from build123d import *

# Parameters (mm, degrees)
SKETCH032_W            = 103
SKETCH032_H            = 207
PAD009_DEPTH           = 18
POCKET017_DEPTH        = 16
SKETCH034_W            = 55
SKETCH034_H            = 79
POCKET018_DEPTH        = 16
POCKET019_DEPTH        = 16
LINEARPATTERN002_COUNT = 3
LINEARPATTERN002_PITCH = 24
POCKET020_DEPTH        = 16
POCKET021_DEPTH        = 16
FILLET008_R            = 8
FILLET009_R            = 15
POCKET022_DEPTH        = 5
POCKET022_DEPTH_BACK   = 100


with BuildPart() as part:
    # Sketch032 → Pad009 (new body)
    with BuildSketch(Plane.XY):
        Rectangle(SKETCH032_W, SKETCH032_H)
    extrude(amount=PAD009_DEPTH)

    # Sketch029 (on Face6 of Pad009) → Pocket017 (cut)
    with BuildSketch(Plane(origin=(10, 69, 18), x_dir=(1, 0, 0), z_dir=(0, 0, 1))):
        Polygon((-40, -32), (40, -32), (40, 32), (-40, 32), (-56, 32), (-56, 16), (-40, 16), align=None)
    extrude(amount=-POCKET017_DEPTH, mode=Mode.SUBTRACT)

    # Sketch034 → Pocket018 (cut)
    with BuildSketch(Plane(origin=(-52, 30, 18), x_dir=(0, 1, 0), z_dir=(0, 0, 1))):
        with Locations((-22, -62)):
            Rectangle(SKETCH034_W, SKETCH034_H)
    extrude(amount=-POCKET018_DEPTH, mode=Mode.SUBTRACT)

    # Sketch030 → Pocket019 (cut)
    with BuildSketch(Plane(origin=(25, -90, 18), x_dir=(1, 0, 0), z_dir=(0, 0, 1))):
        with BuildLine():
            Line((-23.5, 11), (23.5, 11))
            Line((23.5, 11), (15.797717, 0))
            Line((15.797717, 0), (23.5, -11))
            Line((23.5, -11), (-23.5, -11))
            ThreePointArc((-23.5, 11), (-34.5, 0), (-23.5, -11))
        make_face()
    pocket019 = extrude(amount=-POCKET019_DEPTH, mode=Mode.SUBTRACT)

    # LinearPattern002: Pocket019 ×3
    with Locations(*[(0, i * LINEARPATTERN002_PITCH, 0) for i in range(1, LINEARPATTERN002_COUNT)]):
        add(pocket019, mode=Mode.SUBTRACT)

    # Sketch031 → Pocket020 (cut)
    with BuildSketch(Plane(origin=(-68, -55, 18), x_dir=(1, 0, 0), z_dir=(0, 0, 1))):
        with BuildLine():
            Line((51.488981, 23.283394), (51.488981, -34.716606))
            Line((51.488981, -34.716606), (46.488981, -34.716606))
            ThreePointArc((27.488981, -34.716606), (36.988981, -44.216606), (46.488981, -34.716606))
            Line((27.488981, -34.716606), (22.488981, -34.716606))
            Line((22.488981, -34.716606), (22.488981, 23.283394))
            Line((22.488981, 23.283394), (51.488981, 23.283394))
        make_face()
    extrude(amount=-POCKET020_DEPTH, mode=Mode.SUBTRACT)

    # Sketch033 → Pocket021 (cut)
    with BuildSketch(Plane(origin=(-60, 120, 18), x_dir=(1, 0, 0), z_dir=(0, 0, 1))):
        with BuildLine():
            ThreePointArc((10.250873, -136.6297), (19.384811, -145.763638), (28.518749, -136.6297))
            Line((28.518749, -136.6297), (28.518749, -47.133303))
            ThreePointArc((28.518749, -47.133303), (19.384811, -37.999364), (10.250873, -47.133303))
            Line((10.250873, -136.6297), (10.250873, -47.133303))
        make_face()
    extrude(amount=-POCKET021_DEPTH, mode=Mode.SUBTRACT)

    # Fillet008
    fillet008_edges = [part.edges().sort_by_distance(p)[0] for p in [
        (-40.615189, 82.000636, 2),
    ]]
    fillet(fillet008_edges, radius=FILLET008_R)

    # Fillet009
    fillet009_edges = [part.edges().sort_by_distance(p)[0] for p in [
        (-46, 93, 2),
    ]]
    fillet(fillet009_edges, radius=FILLET009_R)

    # Sketch035 → Pocket022 (cut, two sides)
    with BuildSketch(Plane(origin=(50, -35, 2), x_dir=(0, 1, 0), z_dir=(0, 0, 1))) as pocket022_sk:
        with BuildLine():
            ThreePointArc((30.448608, -4.073936), (44.198608, -17.823936), (57.948608, -4.073936))
            Line((57.948608, -4.073936), (57.948608, 22.259397))
            ThreePointArc((57.948608, 22.259397), (44.198608, 36.009397), (30.448608, 22.259397))
            Line((30.448608, -4.073936), (30.448608, 22.259397))
        make_face()
    extrude(amount=-POCKET022_DEPTH, mode=Mode.SUBTRACT)
    extrude(pocket022_sk.sketch, amount=POCKET022_DEPTH_BACK, mode=Mode.SUBTRACT)


solid = part.part
Work out the finished part from the listing and answer in its coordinate system (mm). A direction names the side the tool comes from. Give positions to 0.01 mm unless a question says otherwise; leave off trailing zeros. Order: outer loops, then holes, each group sorted by start corner. A loop starts at its lowest first (then second) coordinate and runs counter-clockwise, first axis right, second up. Notation, with made-up numbers: (66, 65) -> (74, 65) arc R10 cw to (74, 83) -> close; hole circle Ø9 at (42.25, 23.5). An arc over 180 degrees is marked (long way). One line per item, written item: value.
Item 1: Find section D-D, the plane y = 5. Give the vertices of the cut face in (x, z).
Answer sheet:
outline: (-51.5, 0) -> (14.65, 0) -> (14.65, 2) -> (-29.5, 2) -> (-29.5, 18) -> (-31.48, 18) -> (-31.48, 10) arc R8 cw to (-39.48, 2) -> (-41.75, 2) arc R8 cw to (-49.75, 10) -> (-49.75, 18) -> (-51.5, 18) -> close
Item 2: Find section C-C, the plane y = 32. Give the vertices of the cut face in (x, z).
Answer sheet:
outline: (-51.5, 0) -> (51.5, 0) -> (51.5, 18) -> (49.5, 18) -> (49.5, 2) -> (-29.5, 2) -> (-29.5, 18) -> (-31.48, 18) -> (-31.48, 10) arc R8 cw to (-39.48, 2) -> (-41.75, 2) arc R8 cw to (-49.75, 10) -> (-49.75, 18) -> (-51.5, 18) -> close
Item 3: Straight lines are drawn through the part: probe 1 along Y at (x, z) = (-20.5, 14); probe 2 along X at (y, z) = (50.5, 15); probe 3 along Y at (x, z) = (35, 15.5). For each, find the intervals that lie inside material, in ascending order.
Answer sheet:
probe 1: -103.5 to -89.72, -31.72 to -19.5, 35.5 to 37, 101 to 103.5
probe 2: -51.5 to -49.75, -31.48 to -30, 50 to 51.5
probe 3: -103.5 to -101, -79 to -77, -55 to -53, -31 to -19.5, 35.5 to 37, 101 to 103.5
Item 4: A tool of negligible diameter and unlimited length cuts with its end or side. For faces 1 (the flat face through (-49.749, 27, 14)), 2 (the flat face through (45, -4.551, 1.6)), 3 (the flat face through (51.5, 63, 9)), from which of +Z, -Z, +X, -X, +Y, -Y can it reach the whole face along a straight path? Write none if from no direction.
Answer sheet:
face 1: +Z
face 2: +Z, -Z, +X
face 3: +Z, -Z, +X, +Y, -Y
Item 5: Find section A-A, the plane y = 87.5. Give the vertices of the cut face in (x, z), plus the area to 3 significant figures.
Answer sheet:
outline: (-51.5, 0) -> (51.5, 0) -> (51.5, 18) -> (50, 18) -> (50, 2) -> (-31, 2) arc R15 cw to (-46, 17) -> (-46, 18) -> (-51.5, 18) -> close
area: 366 mm²
Item 6: A flat-ended cylindrical pin translates along its axis: P1, Ø0.7, axis at x = -40, y = 32, coming from the +Z side. Find the tip coordinate at first contact, or state that the pin passes through.
Answer sheet:
P1: z = 2
Item 7: Find section B-B, the plane z = 14.5. State how many separate pieces and enclosed holes the cut face has, plus the area to 3 significant figures.
Answer sheet:
separate pieces: 1
enclosed holes: 6
area: 4,410 mm²
Item 8: Determine the mould class of faces 4 (the flat face through (-8, -30, 18)), 5 (the flat face through (-1, 103.5, 9)), 6 (the flat face through (45, -60, 10)) for opening direction Y: released by +Y, released by -Y, zero draft, split by the parting line, or undercut.
Answer sheet:
face 4: zero draft
face 5: released by +Y
face 6: undercut
